Here's how the part is built. I have some questions about the finished solid (model axes, mm). Round coordinates to 2 decimals unless told otherwise and drop trailing zeros. Order: outer loops, then holes, each group sorted by start corner. A loop starts at its lowest first (then second) coordinate and runs counter-clockwise, first axis right, second up. Notation, with made-up numbers: M 15.5,-38.5 L 39.5,-38.5 A21 ccw 39.5,-27.5 Z; hole C -22,9 d11. An arc over 180 degrees is marked long. Write item = value, one per line. Start each with the question number.
Item 1: I'm going to push flat-ended pins straight in: P1, Ø1.8, axis at x = 187.5, z = -1.5, coming from the +Y side; P2, Ø1.8, axis at x = 88, z = -0.5, coming from the +Y side; P3, Ø6, axis at x = 40, z = 0, coming from the +Y side. Where does each tip first touch, or does it pass through?
Item 2: Please list where these lines run through material, in increasing order: L1, parallel to Y at x = 41.5, z = 4.75; L2, parallel to Z at x = 12.5, y = -2; L3, parallel to Z at x = -137.5, y = 1.9.
Item 3: I want a section at A-A, the plane y = -2. State how many separate pieces and enclosed holes the cut face has, plus the area to 3 significant figures.
Item 4: I want a section at B-B, the plane x = -75. List the corners of the cut face in (y, z) for me.
```python
from build123d import *

# Parameters (mm, degrees)
SKETCH_1_W                   = 400
SKETCH_1_H                   = 12
EXTRUDE_1_DEPTH              = 8
CUT_EXTRUDE_1_DEPTH          = 401.06499472
CUT_EXTRUDE_2_DEPTH          = 401.06499472
CUT_EXTRUDE_3_DEPTH          = 401.06499472
CUT_EXTRUDE_4_DEPTH          = 401.06499472
CUT_EXTRUDE_5_DEPTH          = 401.06499472
CUT_EXTRUDE_6_DEPTH          = 401.06499472
HOLE_WIZARD_M3_1_D           = 3.5
HOLE_WIZARD_M3_1_CBORE_D     = 5.9999
HOLE_WIZARD_M3_1_CBORE_DEPTH = 4.5
CHAMFER_1_SIZE               = 0.6
FILLET_1_R                   = 0.2


with BuildPart() as part:
    # 草图1 → 凸台-拉伸1 (new body)
    with BuildSketch(Plane(origin=(0, 4, 0), x_dir=(1, 0, 0), z_dir=(0, 1, 0))):
        Rectangle(SKETCH_1_W, SKETCH_1_H)
    extrude(amount=-EXTRUDE_1_DEPTH)

    # 草图2 → 切除-拉伸1 (cut, through all)
    with BuildSketch(Plane(origin=(200, 0, 0), x_dir=(0, 0, -1), z_dir=(1, 0, 0))):
        with BuildLine():
            Line((6, 1.51), (6, 2.01))
            Line((6, 2.01), (4.8, 2.01))
            ThreePointArc((4.8, 2.01), (4.55, 1.76), (4.8, 1.51))
            Line((4.8, 1.51), (6, 1.51))
        make_face()
    extrude(amount=-CUT_EXTRUDE_1_DEPTH, mode=Mode.SUBTRACT)

    # 草图3 → 切除-拉伸2 (cut, through all)
    with BuildSketch(Plane(origin=(200, 0, 0), x_dir=(0, 0, -1), z_dir=(1, 0, 0))):
        with BuildLine():
            Line((6, 2.01), (6, 3.111111))
            ThreePointArc((6, 3.111111), (5.367595703, 2.693428684), (5.04, 2.01))
            Line((5.04, 2.01), (6, 2.01))
        make_face()
    extrude(amount=-CUT_EXTRUDE_2_DEPTH, mode=Mode.SUBTRACT)

    # 草图4 → 切除-拉伸3 (cut, through all)
    with BuildSketch(Plane(origin=(200, 0, 0), x_dir=(0, 0, -1), z_dir=(1, 0, 0))):
        with BuildLine():
            Line((6, 1.51), (5.04, 1.51))
            ThreePointArc((5.04, 1.51), (5.367595703, 0.826571316), (6, 0.408889))
            Line((6, 0.408889), (6, 1.51))
        make_face()
    extrude(amount=-CUT_EXTRUDE_3_DEPTH, mode=Mode.SUBTRACT)

    # 草图5 → 切除-拉伸4 (cut, through all)
    with BuildSketch(Plane(origin=(200, 0, 0), x_dir=(0, 0, -1), z_dir=(1, 0, 0))):
        with BuildLine():
            Line((-6, 2.01), (-6, 1.51))
            Line((-6, 1.51), (-4.8, 1.51))
            ThreePointArc((-4.8, 1.51), (-4.55, 1.76), (-4.8, 2.01))
            Line((-4.8, 2.01), (-6, 2.01))
        make_face()
    extrude(amount=-CUT_EXTRUDE_4_DEPTH, mode=Mode.SUBTRACT)

    # 草图6 → 切除-拉伸5 (cut, through all)
    with BuildSketch(Plane(origin=(200, 0, 0), x_dir=(0, 0, -1), z_dir=(1, 0, 0))):
        with BuildLine():
            Line((-6, 1.51), (-6, 0.408889))
            ThreePointArc((-6, 0.408889), (-5.367595703, 0.826571316), (-5.04, 1.51))
            Line((-5.04, 1.51), (-6, 1.51))
        make_face()
    extrude(amount=-CUT_EXTRUDE_5_DEPTH, mode=Mode.SUBTRACT)

    # 草图7 → 切除-拉伸6 (cut, through all)
    with BuildSketch(Plane(origin=(200, 0, 0), x_dir=(0, 0, -1), z_dir=(1, 0, 0))):
        with BuildLine():
            Line((-6, 2.01), (-5.04, 2.01))
            ThreePointArc((-5.04, 2.01), (-5.367595703, 2.693428684), (-6, 3.111111))
            Line((-6, 3.111111), (-6, 2.01))
        make_face()
    extrude(amount=-CUT_EXTRUDE_6_DEPTH, mode=Mode.SUBTRACT)

    # M3 六角头机械螺钉的柱形沉头孔1 (through all)
    with Locations(Plane(origin=(0, 4, 0), x_dir=(1, 0, 0), z_dir=(0, 1, 0))):
        with Locations((-187.5, 0), (-162.5, 0), (-137.5, 0), (-112.5, 0), (-87.5, 0), (-62.5, 0), (-37.5, 0), (-12.5, 0), (12.5, 0), (37.5, 0), (62.5, 0), (87.5, 0), (112.5, 0), (137.5, 0), (162.5, 0), (187.5, 0)):
            CounterBoreHole(HOLE_WIZARD_M3_1_D / 2, HOLE_WIZARD_M3_1_CBORE_D / 2, HOLE_WIZARD_M3_1_CBORE_DEPTH)

    # 倒角1
    chamfer_1_edges = [part.edges().sort_by_distance(p)[0] for p in [
        (0, -4, -6),
        (0, -4, 6),
    ]]
    chamfer(chamfer_1_edges, length=CHAMFER_1_SIZE)

    # 圆角1
    fillet_1_edges = [part.edges().sort_by_distance(p)[0] for p in [
        (0, 2.01, -5.04),
        (0, 3.111111, -6),
        (0, 0.408889, -6),
        (0, 1.51, -5.04),
        (0, 4, -6),
        (0, 4, 6),
        (0, 1.51, 5.04),
        (0, 0.408889, 6),
        (0, 3.111111, 6),
        (0, 2.01, 5.04),
    ]]
    fillet(fillet_1_edges, radius=FILLET_1_R)


solid = part.part
```
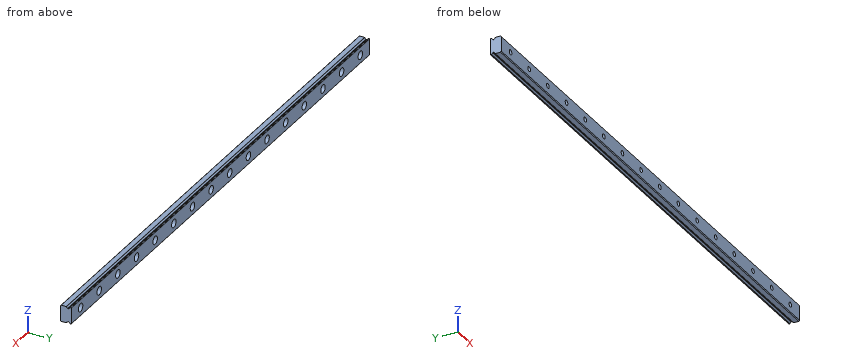
Filled in:
q1.P1 = -0.5
q1.P2 = through
q1.P3 = 4
q2.L1 = -4 to 1.52, 2 to 4
q2.L2 = -6 to -1.75, 1.75 to 6
q2.L3 = -4.59 to -3, 3 to 4.59
q3.separate_pieces = 1
q3.enclosed_holes = 16
q3.area = 4,650 mm^2
q4.outline = M -4,-5.4 L -3.4,-6 L 0.27,-6 A0.2 ccw 0.45,-5.88 A1.42 cw 1.37,-5.07 A0.2 ccw 1.51,-4.88 L 1.51,-4.8 A0.25 cw 2.01,-4.8 L 2.01,-4.88 A0.2 ccw 2.15,-5.07 A1.42 cw 3.07,-5.88 A0.2 ccw 3.25,-6 L 3.8,-6 A0.2 ccw 4,-5.8 L 4,5.8 A0.2 ccw 3.8,6 L 3.25,6 A0.2 ccw 3.07,5.88 A1.42 cw 2.15,5.07 A0.2 ccw 2.01,4.88 L 2.01,4.8 A0.25 cw 1.51,4.8 L 1.51,4.88 A0.2 ccw 1.37,5.07 A1.42 cw 0.45,5.88 A0.2 ccw 0.27,6 L -3.4,6 L -4,5.4 Z
